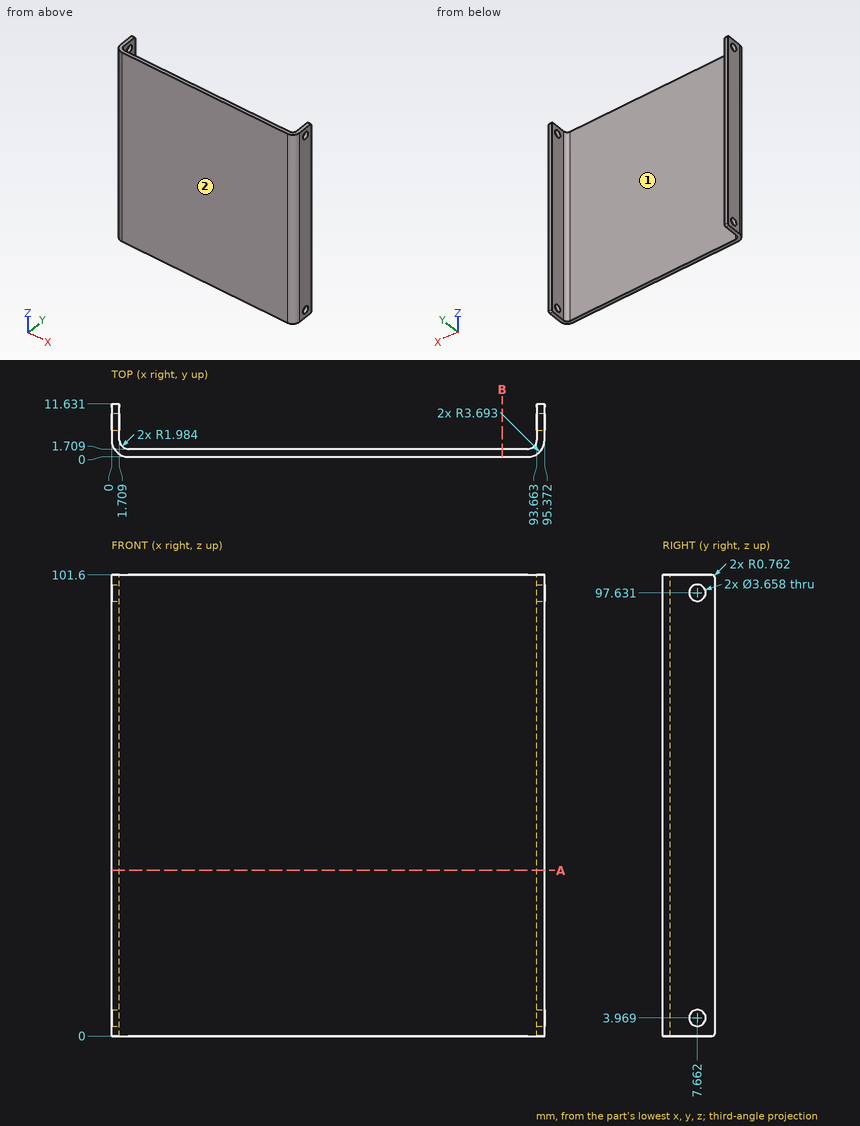
Source: three-view drawing plus pictorial views. Frame: mm from the lowest corner of the part. A direction names the side the tool comes from. Round coordinates to 2 decimals unless told otherwise and drop trailing zeros. Write each loop counter-clockwise with the first axis right and the second up, starting at its lowest first coordinate (ties: lowest second). Pieces come first, ordered by that corner, then holes. Notation, with made-up numbers: M -3,14.25 L 22,14.25 A18 cw 22,39.25 Z; hole C -10,-27 d5. An arc over 180 degrees is marked long. Write item = value, one per line.
Item 1: Access query for the marked faces 1 and 2. Directions: +Z, -Z, +X, -X, +Y, -Y. A direction counts if a zero-diameter tool reaches every point of the face in a straight line with its end or side. Return the directions, or none.
Findings:
face_1 = +Z, -Z, +Y
face_2 = +Z, -Z, +X, -X, -Y
Item 2: Section query B-B on x = 86. Return loops of the section in (y, z).
Findings:
outline = M 0,0 L 1.71,0 L 1.71,101.6 L 0,101.6 Z
Item 3: Material intervals for line 1 along X through (y, z) = (5.75, 28); line 2 along Y through (x, z) = (38, 93.5); line 3 along X through (y, z) = (3, 53) (1 decimal), sorted ascending. Write a range as [from, to].
Findings:
line_1 = [0, 1.71], [93.66, 95.37]
line_2 = [0, 1.71]
line_3 = [0.1, 1.8], [93.5, 95.3]
Item 4: Section query A-A on z = 36.5. Return loops of the section in (x, y), then the cut area to 3 significant figures.
Findings:
outline = M 0,3.69 A3.69 ccw 3.69,0 L 91.68,0 A3.69 ccw 95.37,3.69 L 95.37,11.63 L 93.66,11.63 L 93.66,3.69 A1.98 cw 91.68,1.71 L 3.69,1.71 A1.98 cw 1.71,3.69 L 1.71,11.63 L 0,11.63 Z
area = 193 mm^2
